from build123d import *

# Parameters (mm, degrees)
SKETCH_1_W                = 43.5
SKETCH_1_H                = 38
EXTRUDE_1_DEPTH           = 21.5
SKETCH_2_W                = 40.5
SKETCH_2_H                = 20
CUT_EXTRUDE_1_DEPTH       = 39
CUT_EXTRUDE_2_DEPTH       = 22.5
CUT_EXTRUDE_3_DEPTH       = 22.5
HOLE_WIZARD_8_0_8_1_D     = 8
HOLE_WIZARD_8_0_8_1_DEPTH = 1.5
HOLE_WIZARD_2_0_2_1_D     = 2
HOLE_WIZARD_2_0_2_1_DEPTH = 1.5
HOLE_WIZARD_8_0_8_2_D     = 8
HOLE_WIZARD_8_0_8_2_DEPTH = 1.5
HOLE_WIZARD_2_0_2_2_D     = 2
HOLE_WIZARD_2_0_2_2_DEPTH = 1.5
FILLET_1_R                = 1
FILLET_2_R                = 1.5


with BuildPart() as part:
    # 草图1 → 凸台-拉伸1 (new body)
    with BuildSketch(Plane.XZ.offset(20)):
        Rectangle(SKETCH_1_W, SKETCH_1_H)
    extrude(amount=-EXTRUDE_1_DEPTH)

    # 草图2 → 切除-拉伸1 (cut, through all)
    with BuildSketch(Plane.XY.offset(19)):
        with Locations((0, -10)):
            Rectangle(SKETCH_2_W, SKETCH_2_H)
    extrude(amount=-CUT_EXTRUDE_1_DEPTH, mode=Mode.SUBTRACT)

    # 草图3 → 切除-拉伸2 (cut, through all)
    with BuildSketch(Plane(origin=(0, 1.5, 0), x_dir=(-1, 0, 0), z_dir=(0, 1, 0))):
        with BuildLine():
            Line((14.38749457, 19), (-14.38749457, 19))
            ThreePointArc((-14.38749457, 19), (0, 16), (14.38749457, 19))
        make_face()
    extrude(amount=-CUT_EXTRUDE_2_DEPTH, mode=Mode.SUBTRACT)

    # 草图4 → 切除-拉伸3 (cut, through all)
    with BuildSketch(Plane(origin=(0, 1.5, 0), x_dir=(-1, 0, 0), z_dir=(0, 1, 0))):
        with BuildLine():
            Line((-14.38749457, -19), (14.38749457, -19))
            ThreePointArc((14.38749457, -19), (0, -16), (-14.38749457, -19))
        make_face()
    extrude(amount=-CUT_EXTRUDE_3_DEPTH, mode=Mode.SUBTRACT)

    # Ø8.0 (8) 直径孔1
    with Locations(Plane.ZY.offset(-20.25)):
        with Locations((0, -10)):
            Hole(HOLE_WIZARD_8_0_8_1_D / 2, depth=HOLE_WIZARD_8_0_8_1_DEPTH)

    # Ø2.0 (2) 直径孔1
    with Locations(Plane.ZY.offset(-20.25)):
        with Locations((16.6, -3), (16.6, -17), (9.5, -17.5), (9.6, -10), (9.5, -2.5), (-9.5, -2.5), (-16.6, -3), (-16.6, -17), (-9.5, -17.5), (-9.6, -10)):
            Hole(HOLE_WIZARD_2_0_2_1_D / 2, depth=HOLE_WIZARD_2_0_2_1_DEPTH)

    # Ø8.0 (8) 直径孔2
    with Locations(Plane(origin=(-20.25, 0, 0), x_dir=(0, 0, -1), z_dir=(1, 0, 0))):
        with Locations((0, -10)):
            Hole(HOLE_WIZARD_8_0_8_2_D / 2, depth=HOLE_WIZARD_8_0_8_2_DEPTH)

    # Ø2.0 (2) 直径孔2
    with Locations(Plane(origin=(-20.25, 0, 0), x_dir=(0, 0, -1), z_dir=(1, 0, 0))):
        with Locations((-16.6, -3), (-16.6, -17), (-9.5, -17.5), (-9.6, -10), (-9.5, -2.5), (9.5, -2.5), (16.6, -3), (16.6, -17), (9.5, -17.5), (9.6, -10)):
            Hole(HOLE_WIZARD_2_0_2_2_D / 2, depth=HOLE_WIZARD_2_0_2_2_DEPTH)

    # 圆角1
    fillet_1_edges = [part.edges().sort_by_distance(p)[0] for p in [
        (-21, -20, 19),
        (21, -20, -19),
        (-14.38749457, 0.75, 19),
        (14.38749457, 0.75, 19),
        (14.38749457, 0.75, -19),
        (-14.38749457, 0.75, -19),
        (-21, -20, -19),
        (21, -20, 19),
    ]]
    fillet(fillet_1_edges, radius=FILLET_1_R)

    # 圆角2
    fillet_2_edges = [part.edges().sort_by_distance(p)[0] for p in [
        (-21.75, 1.5, 0),
        (21.75, 1.5, 0),
    ]]
    fillet(fillet_2_edges, radius=FILLET_2_R)


solid = part.part
Read the model definition and answer for the solid it produces. Units are mm, in the model's axes. A direction names the side the tool comes from. Coordinates: 2 decimals unless noted, no trailing zeros. Loops run counter-clockwise (first coordinate to the right, second up) from the corner with the lowest first, then second, coordinate; pieces in that order, holes last.
Q1. The mould has two halves that part along Z. Classify faces 1 (the face through (21.3, 1.07, 0.27)), 2 (the face through (-20.99, -19.699, -18.715)), 3 (the face through (-21, -3.1, -10.3)): +Z half, -Z half, draft (parallel to the pull), parting line (faces both ways), or undercut.
Q2. The part is cut by section D-D on z = -6. Write down the section's boundary in (x, y).
Q3. This flat-tipped pin is pushed along its axis until it touches: pin 1 Ø3 at (x, z) = (1.5, -4) entering from -Y. Where does it stop, or does it pass through?
Q4. The part is cut by section C-C on y = -13.25. Write down the section's boundary in (x, z), and give its area (3 significant figures).
Q5. The part is cut by section A-A on z = 0. Write down the section's boundary in (x, y).
Q6. Consider probe 1 along X at (y, z) = (-9.25, 16); probe 2 along Y at (x, z) = (-20.9, -9.5); probe 3 along Y at (x, z) = (-20, -15.5). Determine where each line is inside the solid, lowest interval first.
Q7. The part is cut by section B-B on z = 9.6. Give the number of separate pieces and of enclosed holes in the cut face, and give its area (3 significant figures).
Q8. Which of the six approach directions +Z, -Z, +X, -X, +Y, -Y give full straight-line access (tool end or side, diameter ignored) to faces 4 (the face through (0, 0, 0)), 5 (the face through (-21, -7, 19))?
Results below:
1. face 1: draft
1. face 2: -Z half
1. face 3: undercut
2. outline: (-21.75, -20) - (-20.25, -20) - (-20.25, 0) - (20.25, 0) - (20.25, -20) - (21.75, -20) - (21.75, 0) arc R1.5 ccw to (20.25, 1.5) - (-20.25, 1.5) arc R1.5 ccw to (-21.75, 0) - close
3. pin 1: stops at y = 0
4. outline: (-21.75, -19) - (-20.25, -19) - (-20.25, -2.33) - (-21.75, -2.33) - close; (-21.75, 2.33) - (-20.25, 2.33) - (-20.25, 19) - (-21.75, 19) - close; (20.25, -19) - (21.75, -19) - (21.75, -2.33) - (20.25, -2.33) - close; (20.25, 2.33) - (21.75, 2.33) - (21.75, 19) - (20.25, 19) - close
4. area: 100 mm2
5. outline: (-21.75, -20) - (-20.25, -20) - (-20.25, -14) - (-21.75, -14) - close; (-21.75, -6) - (-20.25, -6) - (-20.25, 0) - (20.25, 0) - (20.25, -6) - (21.75, -6) - (21.75, 0) arc R1.5 ccw to (20.25, 1.5) - (-20.25, 1.5) arc R1.5 ccw to (-21.75, 0) - close; (20.25, -20) - (21.75, -20) - (21.75, -14) - (20.25, -14) - close
6. probe 1: x = -21.75 to -20.25, 20.25 to 21.75
6. probe 2: y = -20 to -18.5, -16.5 to -10.99, -9.01 to -3.5, -1.5 to 1.35
6. probe 3: y = 0 to 1.5
7. separate pieces: 7
7. enclosed holes: 0
7. area: 106 mm2
8. face 4: +Z, -Z, -Y
8. face 5: +Z, +X, -X, +Y, -Y
